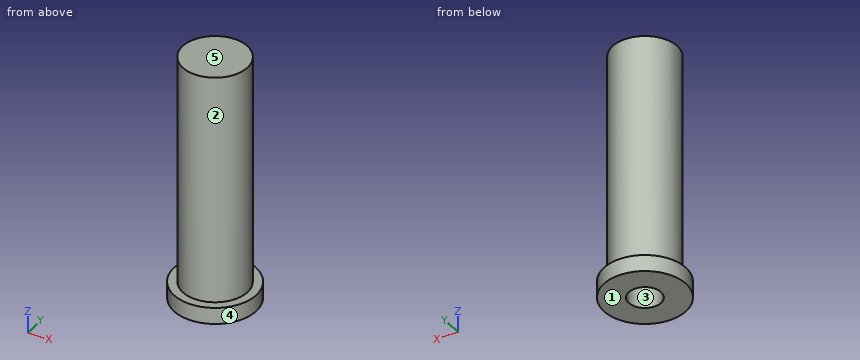
from build123d import *

# Parameters (mm, degrees)
SKETCH2_R               = 5
BOSS_EXTRUDE1_DEPTH     = 35.56
CUT_EXTRUDE1_DEPTH      = 25.4
CUT_EXTRUDE1_DEPTH_BACK = 1
SKETCH3_R               = 6.35
BOSS_EXTRUDE2_DEPTH     = 2.54
CUT_EXTRUDE2_DEPTH      = 2.54
SKETCH5_R               = 2.5
CUT_EXTRUDE3_DEPTH      = 28.575


with BuildPart() as part:
    # Sketch2 → Boss-Extrude1 (new body)
    with BuildSketch(Plane.XY):
        with Locations((13.074576669, 1.623038211)):
            Circle(SKETCH2_R)
    extrude(amount=BOSS_EXTRUDE1_DEPTH)

    # Sketch1 → Cut-Extrude1 (cut, two sides)
    with BuildSketch(Plane.XY) as cut_extrude1_sk:
        with BuildLine():
            Line((15.515382974, 2.163838155), (14.277170381, -0.568711858))
            ThreePointArc((14.277170381, -0.568711858), (10.797451658, 2.654882038), (15.515382974, 2.163838155))
        make_face()
    extrude(amount=CUT_EXTRUDE1_DEPTH, mode=Mode.SUBTRACT)
    extrude(cut_extrude1_sk.sketch, amount=-CUT_EXTRUDE1_DEPTH_BACK, mode=Mode.SUBTRACT)

    # Sketch3 → Boss-Extrude2 (add)
    with BuildSketch(Plane(origin=(0, 0, 0), x_dir=(-1, 0, 0), z_dir=(0, 0, -1))):
        with Locations((-13.074576669, 1.623038211)):
            Circle(SKETCH3_R)
    extrude(amount=BOSS_EXTRUDE2_DEPTH)

    # Sketch4 → Cut-Extrude2 (cut)
    with BuildSketch(Plane(origin=(0, 0, -2.54), x_dir=(-1, 0, 0), z_dir=(0, 0, -1))):
        with BuildLine():
            Line((-15.515382974, 2.163838155), (-14.277170381, -0.568711858))
            ThreePointArc((-14.277170381, -0.568711858), (-10.797451658, 2.654882038), (-15.515382974, 2.163838155))
        make_face()
    extrude(amount=-CUT_EXTRUDE2_DEPTH, mode=Mode.SUBTRACT)

    # Sketch5 → Cut-Extrude3 (cut)
    with BuildSketch(Plane(origin=(0, 0, -2.54), x_dir=(-1, 0, 0), z_dir=(0, 0, -1))):
        with Locations((-13.074576669, 1.623038211)):
            Circle(SKETCH5_R)
    extrude(amount=-CUT_EXTRUDE3_DEPTH, mode=Mode.SUBTRACT)


solid = part.part
CAD build for the part. Positions are in the model's coordinates, mm. Face numbers are marked on the shaded views. A direction names the side the tool comes from. Round coordinates to 2 decimals unless told otherwise and drop trailing zeros. Loops run counter-clockwise (first coordinate to the right, second up) from the corner with the lowest first, then second, coordinate; pieces in that order, holes last. Notation, with made-up numbers: M 28,-37 L 42,-37 A28 ccw 42,-8 Z; hole C 32.25,83.25 d1. An arc over 180 degrees is marked long. One line per question, with ' | ' between items. Start each with the question number.
Item 1: Cut at C-C, the plane z = 12.5. Write the cut outline in (x, y).
Item 2: Cut at B-B, the plane y = -2.5. Write the cut outline in (x, z), plus the area to 3 significant figures.
Item 3: Two-plate mould, pull along X, no slides. Class the marked faces 3, 4 and 5: pulls with the +X half, pulls with the -X half, needs draft (parallel to the pull), parting line crosses it, or undercut.
Item 4: Pin check, flat tips, straight feed: pin 1 Ø3 at (x, z) = (11, 4.5) entering from +Y; pin 2 Ø6 at (x, z) = (18, 30.5) entering from +Y; pin 3 Ø1.5 at (x, y) = (13, 3) entering from -Z (3 decimals). Stop position of each tip, or through.
Item 5: Cut at A-A, the plane x = 16.25. Write the cut outline in (y, z).
Item 6: Cut at D-D, the plane z = 32. Write the cut outline in (x, y).
Item 7: Wall check: line 1 (X direction, y = 1.5, z = 12.5); line 2 (Z direction, x = 12.5, y = -0.5) (3 decimals); line 3 (X direction, y = 3, z = 5). Give the ranges that are in metal, low to high.
Item 8: Which spindle directions (+Z, -Z, +X, -X, +Y, -Y) get a long thin tool onto all of the face, cutting with end or side? Do the marked faces 1 and 2. Say none if no direction does.
Responses:
1) outline: C 13.07,1.62 d10; hole C 13.07,1.62 d5
2) outline: M 8.25,-2.54 L 17.9,-2.54 L 17.9,0 L 15.9,0 L 15.9,35.56 L 10.25,35.56 L 10.25,0 L 8.25,0 Z | area: 226 mm²
3) face 3: undercut | face 4: parting line crosses it | face 5: needs draft
4) pin 1: stops at y = 6.59 | pin 2: stops at y = 6.24 | pin 3: stops at z = 26.035
5) outline: M -3.88,-2.54 L 7.12,-2.54 L 7.12,0 L 5.49,0 L 5.49,35.56 L -2.24,35.56 L -2.24,0 L -3.88,0 Z
6) outline: C 13.07,1.62 d10
7) line 1: x = 8.08 to 10.58, 15.57 to 18.07 | line 2: z = 26.035 to 35.56 | line 3: x = 8.27 to 10.99, 15.16 to 17.88
8) face 1: -Z, +X, -X, +Y, -Y | face 2: +Z
